Autodesk Inventor part; units mm, degrees
ref_plane "YZ Plane" through (0, 0, 0) normal (1, 0, 0) x (0, 1, 0)
ref_plane "XZ Plane" through (0, 0, 0) normal (0, 1, 0) x (-1, 0, 0)
ref_plane "XY Plane" through (0, 0, 0) normal (0, 0, 1) x (1, 0, 0)
sketch "Sketch1" plane through (0, 0, 0) normal (0, 0, 1) x (1, 0, 0)
  point P0 (0, 0)
sketch "Sketch2" plane through (0, 0, 0) normal (0, 0, 1) x (1, 0, 0)
  line L0 (0, 0) -> (-166, 0)
  line L1 (-166, -98.3) -> (0, -98.3)
  line L2 (0, 0) -> (-163, 0)
  line L3 (0, -19.5) -> (0, 0)
  line L4 (-3, 0) -> (0, 0)
  line L5 (0, 0) -> (0, -19.5)
  line L6 (-166, -19.5) -> (-163, -19.5)
  line L7 (-166, -24.5) -> (-163, -24.5)
  line L8 (-166, -98.3) -> (-3, -98.3)
  line L9 (-166, -74.3) -> (-166, -98.3)
  line L10 (-163, -98.3) -> (-166, -98.3)
  line L11 (-166, -98.3) -> (-166, -74.3)
  line L12 (-163, -69.3) -> (-166, -69.3)
  line L13 (-166, -74.3) -> (-163, -74.3)
  arc A0 (-163, -74.3) -> (-163, -69.3) centre (-163, -71.8) ccw
  line L14 (-166, -74.3) -> (-166, -98.3)
  line L15 (-166, 0) -> (-166, -19.5)
  line L16 (-166, -24.5) -> (-166, -69.3)
  line L17 (0, -69.3) -> (-3, -69.3)
  line L18 (-3, -69.3) -> (0, -69.3)
  line L19 (0, -74.3) -> (-3, -74.3)
  arc A1 (-3, -69.3) -> (-3, -74.3) centre (-3, -71.8) ccw
  arc A2 (-163.2703, -24.5) -> (-163.2703, -19.5) centre (-163.2703, -22) ccw
  line L20 (0, -98.3) -> (0, -74.3)
  line L21 (-163.2703, -19.5) -> (-163, -19.5)
  line L22 (-163, -24.5) -> (-163.2703, -24.5)
  line L23 (0, -19.5) -> (-3, -19.5)
  line L24 (-3, -24.5) -> (0, -24.5)
  arc A3 (-3, -19.5) -> (-3, -24.5) centre (-3, -22) ccw
  line L25 (-3.2703, -19.5) -> (-3.2703, -19.5147)
  line L26 (-3.2703, -24.4853) -> (-3.2703, -24.5)
  line L27 (0, -69.3) -> (0, -24.5)
  line L28 (0, -19.5) -> (0, 0)
  dimension "d19" = 160
  dimension "d21" = 49.8
extrude "Extrusion1" add sketch "Sketch2" along normal blind 33.2
sketch "Sketch3" plane through (0, 0, 33.2) normal (0, 0, 1) x (1, 0, 0)
  line L0 (-9, 0) -> (-9, -93.8)
  line L1 (-166, -93.8) -> (-166, 0)
  line L2 (-157, 0) -> (-157, -93.8)
  line L3 (-9, -93.8) -> (-9, 0)
  line L4 (-9, -93.8) -> (0, -93.8)
  line L5 (0, -93.8) -> (0, 0)
  line L6 (0, 0) -> (-9, 0)
  line L7 (-9, 0) -> (-9, -93.8)
  line L8 (-166, 0) -> (-166, -19.5)
  line L9 (-166, 0) -> (-157, 0)
  line L10 (-157, 0) -> (-157, -93.8)
  line L11 (-157, -93.8) -> (-166, -93.8)
  line L12 (-166, -93.8) -> (-166, 0)
  dimension "d24" = 157
  dimension "d25" = 93.8
  dimension "d26" = 148
extrude "Extrusion2" cut sketch "Sketch3" against normal blind 28.7
sketch "Sketch4" plane through (-166, -98.3, 0) normal (0, -1, 0) x (1, 0, 0)
  line L0 (166, 33.2) -> (163, 33.2)
  line L1 (166, 19.3) -> (166, 33.2)
  line L2 (166, 0) -> (166, 33.2)
  line L3 (166, 19.3) -> (163, 19.3)
  line L4 (166, 14.3) -> (163, 14.3)
  arc A0 (163, 19.3) -> (163, 14.3) centre (163, 16.8) ccw
  line L5 (0, 33.2) -> (166, 33.2)
  line L6 (0, 33.2) -> (3, 33.2)
  line L7 (0, 14.3) -> (3, 14.3)
  line L8 (0, 19.3) -> (3, 19.3)
  arc A1 (3, 14.3) -> (3, 19.3) centre (3, 16.8) ccw
  line L9 (0, 19.3) -> (0, 14.3)
  line L10 (0, 0) -> (0, 33.2)
extrude "Extrusion3" cut sketch "Sketch4" against normal blind 28.7
properties part number "Complete Driver"
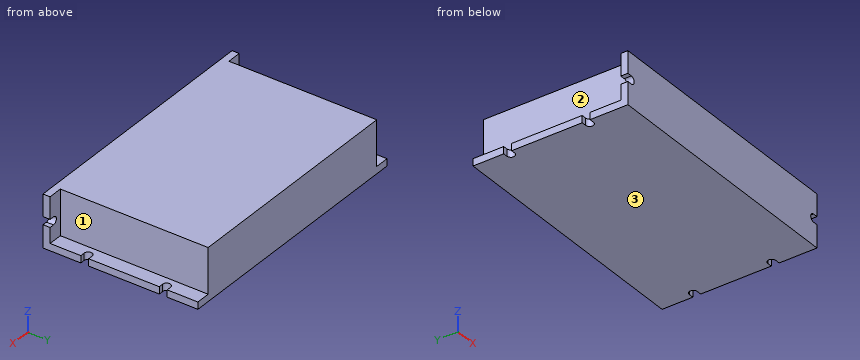
Verification items for the finished model (mm, model axes). Face numbers are marked on the shaded views. A direction names the side the tool comes from. Give positions to 0.01 mm unless a question says otherwise; leave off trailing zeros. Loops run counter-clockwise (first coordinate to the right, second up) from the corner with the lowest first, then second, coordinate; pieces in that order, holes last.
1) Depth check by flat-ended pin: pin 1 Ø8.5 at (y, z) = (-62, 22.5) entering from -X; pin 2 Ø7 at (x, z) = (-162.5, 23) entering from +Y; pin 3 Ø4.5 at (x, y) = (-6, -67) entering from +Z. Enter the tip coordinate at first touch or a pass-through.
2) Sectioned sample at A-A, the plane y = -40.5. Enter the section's corners in (x, z), then the cut area to 3 significant figures.
3) Set-up check for the marked faces 1, 2 and 3: record each of +Z, -Z, +X, -X, +Y, -Y from which the full face is reachable in a straight line by a thin tool's end or side.
4) Thickness scan on line 1 along X through (y, z) = (-19.5, 5). Record the ranges inside material, lowest first.
5) Sectioned sample at B-B, the plane z = 16.8. Enter the section's corners in (x, y).
Answers:
1. pin 1: stops at x = -157
1. pin 2: stops at y = -93.8
1. pin 3: stops at z = 4.5
2. outline: (-166, 0) - (0, 0) - (0, 4.5) - (-9, 4.5) - (-9, 33.2) - (-157, 33.2) - (-157, 4.5) - (-166, 4.5) - close
2. area: 4,990 mm2
3. face 1: +Z, +X, +Y
3. face 2: +Z, -X, +Y
3. face 3: -Z, +X, -X, +Y, -Y
4. line 1: x = -157 to -9
5. outline: (-160.5, -98.3) - (-5.5, -98.3) - (-5.5, -93.8) - (-9, -93.8) - (-9, 0) - (-157, 0) - (-157, -93.8) - (-160.5, -93.8) - close
